Geometry check sheet. Reference: the model listing, model coordinates, mm. A direction names the side the tool comes from. Coordinates: 2 decimals unless noted, no trailing zeros. Write each loop counter-clockwise with the first axis right and the second up, starting at its lowest first coordinate (ties: lowest second). Pieces come first, ordered by that corner, then holes. Notation, with made-up numbers: (-18.5, -26) -> (9.5, -26) arc R24 cw to (9.5, -7) -> close; hole circle Ø8 at (-27.5, 39). An arc over 180 degrees is marked (long way). Answer in a Markdown table with one row per item. Add a question column.
1. Set-up check for faces 1 (the flat face through (48.572, 13, -31)), 2 (the flat face through (27.34, -37.57, -12.41)): record each of +Z, -Z, +X, -X, +Y, -Y from which the full face is reachable in a straight line by a thin tool's end or side.
2. Cross-section at B-B on y = 16. Record the cut outline in (x, z), and give its area (3 significant figures).
3. Cross-section at A-A on x = -28. Record the cut outline in (y, z).
4. Cross-section at D-D on y = -53. Record the cut outline in (x, z).
5. Cross-section at C-C on z = -31.5. Record the cut outline in (x, y).
6. Scan lines: L1, parallel to X at y = -51.5, z = 23; L2, parallel to Z at x = -43.5, y = -30.5; L3, parallel to X at y = -50.5, z = -11.5. Record each from-to range of solid material in increasing order. Write a range as from..to.
7. Mould release check, pull along Y, two halves, no side actions. Record for faces 3 (the flat face through (-11, -76.2, -11)), 4 (the flat face through (-5.697, -42.226, -11.176)), 5 (the flat face through (-11, 25.4, 1)), 6 (the flat face through (-28, -38, 32.139)): pulls with the +Y half, pulls with the -Y half, needs draft (parallel to the pull), parting line crosses it, or undercut.
8. Depth check by flat-ended pin: P1, Ø12.5, axis at x = -29.5, y = -24, coming from the +Z side; P2, Ø2, axis at x = 2.5, y = -50.5, coming from the +Z side; P3, Ø3, axis at y = -43.5, z = 25, coming from the +X side. Enter the tip coordinate at first touch or a pass-through.
```python
from build123d import *

# Parameters (mm, degrees)
F1_DEPTH = 76.2
F2_DEPTH = 25.4
F3_R     = 18.658433191
F4_DEPTH = 25.4


with BuildPart() as f1:
    # F0 (on Front) → F1 (new body)
    with BuildSketch(Plane.XZ):
        Polygon((-7.0377709532, 32.1391718601), (-48.5718883574, 32.1391718601), (-48.5718883574, -39.9264059961), (48.5718883574, -39.9264059961), align=None)
    extrude(amount=F1_DEPTH)

    # F0 (on Front) → F2 (join)
    with BuildSketch(Plane.XZ):
        Polygon((48.5718883574, -21.0635364056), (1.5087825138, 39.9264059961), (-48.5718883574, 39.9264059961), (-48.5718883574, 32.1391718601), (-7.0377709532, 32.1391718601), (48.5718883574, -39.9264059961), align=None)
        Polygon((-7.0377709532, 32.1391718601), (-48.5718883574, 32.1391718601), (-48.5718883574, -39.9264059961), (48.5718883574, -39.9264059961), align=None)
    extrude(amount=-F2_DEPTH)

    # F3 (on face) → F4 (cut)
    with BuildSketch(Plane(origin=(11.1332502223, 0, 8.5910121073), x_dir=(0, 1, 0), z_dir=(0.7916961056, 0, 0.6109151139))):
        with Locations((-41.9644452631, -5.6286053732)):
            Circle(F3_R)
    extrude(amount=-F4_DEPTH, mode=Mode.SUBTRACT)


solid = f1.part
```
Results found:
| question | item | result |
|---|---|---|
| 1 | face 1 | +Z, -Z, +X, +Y, -Y |
| 1 | face 2 | +Z, +X, -Y |
| 2 | outline | (-48.57, -39.93) -> (48.57, -39.93) -> (48.57, -21.06) -> (1.51, 39.93) -> (-48.57, 39.93) -> close |
| 2 | area | 6,320 mm^2 |
| 3 | outline | (-76.2, -39.93) -> (25.4, -39.93) -> (25.4, 39.93) -> (0, 39.93) -> (0, 32.14) -> (-76.2, 32.14) -> close |
| 4 | outline | (-48.57, -39.93) -> (48.57, -39.93) -> (23.76, -7.78) -> (3.65, -23.29) -> (-14.73, 0.53) -> (5.38, 16.05) -> (-7.04, 32.14) -> (-48.57, 32.14) -> close |
| 5 | outline | (-48.57, -76.2) -> (42.07, -76.2) -> (42.07, 0) -> (48.57, 0) -> (48.57, 25.4) -> (-48.57, 25.4) -> close |
| 6 | L1 | x = -48.57..0.01 |
| 6 | L2 | z = -39.93..32.14 |
| 6 | L3 | x = -48.57..-5.45, 21.47..26.64 |
| 7 | face 3 | pulls with the -Y half |
| 7 | face 4 | undercut |
| 7 | face 5 | pulls with the +Y half |
| 7 | face 6 | needs draft |
| 8 | P1 | stops at z = 32.14 |
| 8 | P2 | stops at z = 21.07 |
| 8 | P3 | stops at x = -0.37 |
